Check sheet for the modelled part. Datum: model origin and axes. Units: mm. Round coordinates to 2 decimals unless told otherwise and drop trailing zeros. Write each loop counter-clockwise with the first axis right and the second up, starting at its lowest first coordinate (ties: lowest second). Pieces come first, ordered by that corner, then holes. Notation, with made-up numbers: (82.5, 35) -> (100.5, 35) arc R25 cw to (100.5, 58) -> close; hole circle Ø10 at (46, 1). An arc over 180 degrees is marked (long way). Write item = value, one per line.
from build123d import *

# Parameters (mm, degrees)
SKETCH_1_W           = 120
SKETCH_1_H           = 15
EXTRUDE_1_DEPTH      = 8
FILLET_1_R           = 5
SKETCH_6_R           = 12.5
EXTRUDE_2_DEPTH      = 8
SKETCH_9_W           = 8
SKETCH_9_H           = 15
EXTRUDE_3_DEPTH      = 100
FILLET_2_R           = 10
FILLET_4_R           = 5
SKETCH_11_R          = 1
CUT_EXTRUDE_8_DEPTH  = 10
EXTRUDE_5_DEPTH      = 20
EXTRUDE_5_DEPTH_BACK = 25
SKETCH_15_R          = 3
SKETCH_16_R          = 12.5
EXTRUDE_6_DEPTH      = 5
EXTRUDE_START        = 5
SKETCH_17_R          = 12.5
EXTRUDE_7_DEPTH      = 5


with BuildPart() as part:
    # 草图1 → 凸台-拉伸1 (new body)
    with BuildSketch(Plane(origin=(0, 0, 0), x_dir=(0, 0, -1), z_dir=(1, 0, 0))):
        with Locations((60, 7.5)):
            Rectangle(SKETCH_1_W, SKETCH_1_H)
    extrude(amount=EXTRUDE_1_DEPTH)

    # 圆角1
    fillet_1_edges = [part.edges().sort_by_distance(p)[0] for p in [
        (4, 15, 0),
        (4, 15, -120),
        (4, 0, -120),
        (4, 0, 0),
    ]]
    fillet(fillet_1_edges, radius=FILLET_1_R)

    # 草图6 → 凸台-拉伸2 (add)
    with BuildSketch(Plane(origin=(8, 0, 0), x_dir=(0, 0, -1), z_dir=(1, 0, 0))):
        with Locations((6.4, 7.5)):
            Circle(SKETCH_6_R)
    extrude(amount=-EXTRUDE_2_DEPTH)

    # 草图9 → 凸台-拉伸3 (add)
    with BuildSketch(Plane.XY):
        with Locations((4, 7.5)):
            Rectangle(SKETCH_9_W, SKETCH_9_H)
    extrude(amount=EXTRUDE_3_DEPTH)

    # 圆角2
    fillet_2_edges = [part.edges().sort_by_distance(p)[0] for p in [
        (4, 0, -16.4),
        (4, 15, -16.4),
        (4, 15, 3.6),
        (4, 0, 3.6),
    ]]
    fillet(fillet_2_edges, radius=FILLET_2_R)

    # 圆角4
    fillet_4_edges = [part.edges().sort_by_distance(p)[0] for p in [
        (4, 0, 100),
        (4, 15, 100),
    ]]
    fillet(fillet_4_edges, radius=FILLET_4_R)

    # 草图11 → 切除-拉伸8 (cut)
    with BuildSketch(Plane.ZY):
        with Locations((-115, 7.5)):
            Circle(SKETCH_11_R)
        with Locations((-105, 7.5)):
            Circle(SKETCH_11_R)
        with Locations((85, 7.5)):
            Circle(SKETCH_11_R)
        with Locations((95, 7.5)):
            Circle(SKETCH_11_R)
    extrude(amount=-CUT_EXTRUDE_8_DEPTH, mode=Mode.SUBTRACT)

    # 草图15 → 凸台-拉伸5 (add, two sides: drawn at the far end of the back side and taken through both)
    with BuildSketch(Plane.ZY.offset(-EXTRUDE_5_DEPTH_BACK)):
        with Locations((-6.4, 7.5)):
            Circle(SKETCH_15_R)
    extrude(amount=EXTRUDE_5_DEPTH + EXTRUDE_5_DEPTH_BACK)

    # 草图16 → 凸台-拉伸6 (add)
    with BuildSketch(Plane.ZY.offset(20)):
        with Locations((-6.4, 7.5)):
            Circle(SKETCH_16_R)
    extrude(amount=EXTRUDE_6_DEPTH)

    # 草图17 → 凸台-拉伸7 (add)
    with BuildSketch(Plane(origin=(25, 0, 0), x_dir=(0, 0, -1), z_dir=(1, 0, 0)).offset(EXTRUDE_START)):
        with Locations(Location((6.4, 7.5, 0), (0, 0, 180))):
            Circle(SKETCH_17_R)
    extrude(amount=-EXTRUDE_7_DEPTH)


solid = part.part
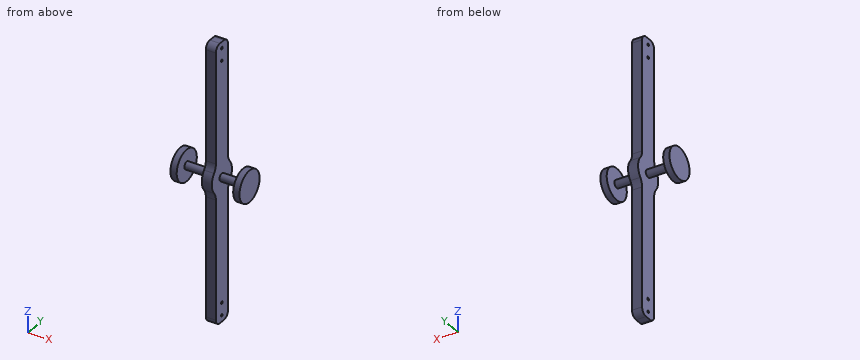
(1) Sectioned sample at C-C on z = 70.5. Enter the section's corners in (x, y), then the cut area to 3 significant figures.
Worked answers:
outline = (0, 0) -> (8, 0) -> (8, 15) -> (0, 15) -> close
area = 120 mm²
(2) Sectioned sample at A-A on z = -6.4. Enter the section's corners in (x, y), then the cut area to 3 significant figures.
Worked answers:
outline = (-25, -5) -> (-20, -5) -> (-20, 4.5) -> (0, 4.5) -> (0, -5) -> (8, -5) -> (8, 4.5) -> (25, 4.5) -> (25, -5) -> (30, -5) -> (30, 20) -> (25, 20) -> (25, 10.5) -> (8, 10.5) -> (8, 20) -> (0, 20) -> (0, 10.5) -> (-20, 10.5) -> (-20, 20) -> (-25, 20) -> close
area = 672 mm²
(3) Go/stop test with flat-tipped pins: P1, Ø3, axis at y = 7.5, z = 85, coming from the -X side; P2, Ø9, axis at x = 2.5, z = -65, coming from the +Y side; P3, Ø1, axis at y = 13.5, z = -20, coming from the +X side; P4, Ø1.8, axis at y = 7.5, z = -115, coming from the -X side. Record where each tip stops, or that it passes through.
Worked answers:
P1 = 0
P2 = 15
P3 = 8
P4 = through
(4) Sectioned sample at B-B on x = -10.5. Enter the section's corners in (y, z), then the cut area to 3 significant figures.
Worked answers:
outline = circle Ø6 at (7.5, -6.4)
area = 28.3 mm²
(5) Material ranges on L1, parallel to X at y = -0.5, z = -2; L2, parallel to Y at x = 4.5, z = -105; L3, parallel to Z at x = 6.5, y = 6.75, recorded low to high. Write a range as [from, to].
Worked answers:
L1 = [-25, -20], [0, 8], [25, 30]
L2 = [0, 6.5], [8.5, 15]
L3 = [-120, -115.66], [-114.34, -105.66], [-104.34, 84.34], [85.66, 94.34], [95.66, 100]
